Source: CAD feature listing. Evaluate the final solid. Frame: model axes, mm. Face numbers are marked on the shaded views. A direction names the side the tool comes from. Coordinates: 2 decimals unless noted, no trailing zeros. Write each loop counter-clockwise with the first axis right and the second up, starting at its lowest first coordinate (ties: lowest second). Pieces come first, ordered by that corner, then holes. Notation, with made-up numbers: (-2, -23.75) - (20, -23.75) arc R25 ccw to (20, 2.25) - close; hole circle Ø9 at (62, -38.5). An arc over 180 degrees is marked (long way). One line per item, written item: value.
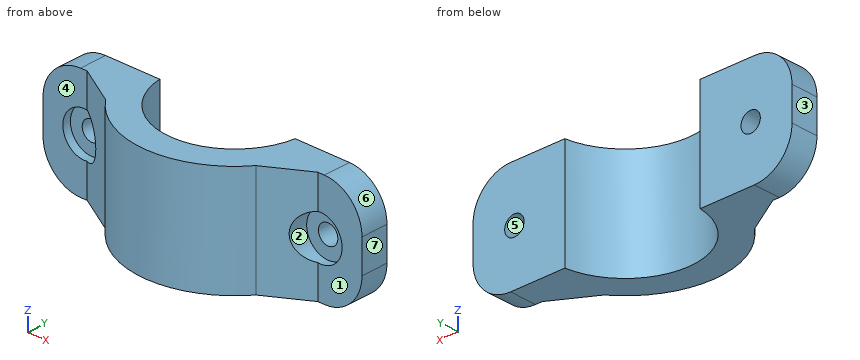
from build123d import *

# Parameters (mm, degrees)
CYLINDER001_R     = 4
CYLINDER001_DEPTH = 20
CYLINDER_R        = 1.8
CYLINDER_DEPTH    = 20
ARRAY_X_COUNT     = 2
ARRAY_X_PITCH     = 44
PAD_DEPTH         = 20
PAD001_DEPTH      = 5


with BuildPart() as bolt_head_hole:
    # Cylinder001 → Cylinder001 (new body)
    with BuildSketch(Plane.XZ):
        Circle(CYLINDER001_R)
    extrude(amount=CYLINDER001_DEPTH)


with BuildPart() as bolt_hole_array:
    # Cylinder → Cylinder (new body)
    with BuildSketch(Plane.XZ.offset(-10)):
        Circle(CYLINDER_R)
    extrude(amount=CYLINDER_DEPTH)

    # Fusion: union bolt head hole
    add(bolt_head_hole.part)

    # Array X: bolt hole array ×2


with BuildPart() as bolt_hole_array_1:
    add(bolt_hole_array.part)
    with Locations(*[(i * ARRAY_X_PITCH, 0, 0) for i in range(1, ARRAY_X_COUNT)]):
        add(bolt_hole_array.part)


with BuildPart() as bolt_hole_array_2:
    # Array placement: moved
    add(bolt_hole_array_1.part.moved(Location((-22, -5, 10))))


with BuildPart() as f_25_mm_attachment_body:
    # Sketch → Pad (new body)
    with BuildSketch(Plane.XY):
        with BuildLine():
            ThreePointArc((12.611106, 1.5), (0, 12.7), (-12.611106, 1.5))
            Line((-22.7, 1.5), (-12.611106, 1.5))
            Line((-22.7, 1.5), (-22.7, 6.5))
            Line((-22.7, 6.5), (-21.463293, 6.5))
            Line((-21.463293, 6.5), (-13.988671, 10.84468))
            ThreePointArc((13.988671, 10.84468), (0, 17.7), (-13.988671, 10.84468))
            Line((13.988671, 10.84468), (21.463293, 6.5))
            Line((21.463293, 6.5), (22.7, 6.5))
            Line((22.7, 6.5), (22.7, 1.5))
            Line((12.611106, 1.5), (22.7, 1.5))
        make_face()
    extrude(amount=PAD_DEPTH)

    # Sketch001 → Pad001 (join)
    with BuildSketch(Plane.XZ.offset(-1.5)):
        with BuildLine():
            Line((-12.611106, 20), (-22.7, 20))
            ThreePointArc((-22.7, 20), (-27.649747, 17.949747), (-29.7, 13))
            Line((-29.7, 13), (-29.7, 7))
            ThreePointArc((-29.7, 7), (-27.649747, 2.050253), (-22.7, 0))
            Line((-12.611106, 0), (-22.7, 0))
            Line((-12.611106, 20), (-12.611106, 0))
        make_face()
        with BuildLine():
            Line((12.611106, 20), (22.7, 20))
            ThreePointArc((29.7, 13), (27.649747, 17.949747), (22.7, 20))
            Line((29.7, 13), (29.7, 7))
            ThreePointArc((22.7, 0), (27.649747, 2.050253), (29.7, 7))
            Line((22.7, 0), (12.611106, 0))
            Line((12.611106, 20), (12.611106, 0))
        make_face()
    extrude(amount=-PAD001_DEPTH)


with BuildPart() as f_25_mm_attachment_holed_clone:
    # Part__Mirroring: instance of 25 mm attachment body
    add(f_25_mm_attachment_body.part.mirror(Plane(origin=(0, 0, 0), x_dir=(1, 0, 0), z_dir=(0, 1, 0))))

    # Cut: cut bolt hole array
    add(bolt_hole_array_2.part, mode=Mode.SUBTRACT)


solid = f_25_mm_attachment_holed_clone.part
1) Draft query along Z for the marked faces 5, 6 and 7. Return one class per face: released by +Z, released by -Z, zero draft, split by the parting line, or undercut.
Values found:
face 5: undercut
face 6: released by +Z
face 7: zero draft
2) Section query D-D on z = 18. Output: boundary loops of the cut face in (x, y), then the cut area to 3 significant figures.
Values found:
outline: (-27.6, -6.5) - (-21.46, -6.5) - (-13.99, -10.84) arc R17.7 ccw to (13.99, -10.84) - (21.46, -6.5) - (27.6, -6.5) - (27.6, -1.5) - (12.61, -1.5) arc R12.7 cw to (-12.61, -1.5) - (-27.6, -1.5) - close
area: 348 mm2
3) Section query B-B on x = -22. Output: boundary loops of the cut face in (y, z).
Values found:
outline: (-6.5, 0) - (-1.5, 0) - (-1.5, 8.2) - (-5, 8.2) - (-5, 6) - (-6.5, 6) - close; (-6.5, 14) - (-5, 14) - (-5, 11.8) - (-1.5, 11.8) - (-1.5, 20) - (-6.5, 20) - close
4) Reachability of the marked faces 1, 2, 3 and 4 from +Z, -Z, +X, -X, +Y, -Y: full face, straight path, thin tool, end or side. Return the list, or none.
Values found:
face 1: +Z, -Z, +X, -Y
face 2: -Y
face 3: +Z, -Z, -X, +Y, -Y
face 4: +Z, -Z, -X, -Y
5) Section query A-A on z = 10. Output: boundary loops of the cut face in (x, y).
Values found:
outline: (-29.7, -6.5) - (-26, -6.5) - (-26, -5) - (-23.8, -5) - (-23.8, -1.5) - (-29.7, -1.5) - close; (-20.2, -5) - (-18, -5) - (-18, -8.51) - (-13.99, -10.84) arc R17.7 ccw to (13.99, -10.84) - (18, -8.51) - (18, -5) - (20.2, -5) - (20.2, -1.5) - (12.61, -1.5) arc R12.7 cw to (-12.61, -1.5) - (-20.2, -1.5) - close; (23.8, -5) - (26, -5) - (26, -6.5) - (29.7, -6.5) - (29.7, -1.5) - (23.8, -1.5) - close
6) Contact query for flat-ended pins moving along their axis: P1, Ø4, axis at x = 25.5, z = 5, coming from the -Y side; P2, Ø3, axis at x = 10.5, z = 15.5, coming from the -Y side; P3, Ø1.5, axis at y = -7, z = 17.5, coming from the -X side; P4, Ø2, axis at x = -22, z = 10, coming from the -Y side. Output: stop coordinate, or through.
Values found:
P1: y = -6.5
P2: y = -15.24
P3: x = -28.49
P4: through
7) Section query C-C on y = -3.5. Output: boundary loops of the cut face in (x, z).
Values found:
outline: (-29.7, 7) arc R7 ccw to (-22.7, 0) - (-12.21, 0) - (-12.21, 20) - (-22.7, 20) arc R7 ccw to (-29.7, 13) - close; (12.21, 0) - (22.7, 0) arc R7 ccw to (29.7, 7) - (29.7, 13) arc R7 ccw to (22.7, 20) - (12.21, 20) - close; hole circle Ø3.6 at (-22, 10); hole circle Ø3.6 at (22, 10)
8) Material intervals for line 1 (Z direction, x = -22, y = -5.8); line 2 (X direction, y = -3.1, z = 10); line 3 (Z direction, x = 22, y = -2.25), sorted ascending.
Values found:
line 1: 0 to 6, 14 to 20
line 2: -29.7 to -23.8, -20.2 to -12.32, 12.32 to 20.2, 23.8 to 29.7
line 3: 0 to 8.2, 11.8 to 20
